```python
from build123d import *

# Parameters (mm, degrees)
F2_R     = 4.7625
F3_DEPTH = 9.525
F4_R     = 1.5875
F5_DEPTH = 22.225


with BuildPart() as f1:
    # F0 (on Front) → F1 (revolve)
    with BuildSketch(Plane.XZ):
        with BuildLine():
            Line((0, 60.744923), (0, 0))
            Line((0, 0), (13.365728, 15.209274))
            ThreePointArc((13.365728, 15.209274), (21.391858, 21.354408), (31.158879, 23.959541))
            ThreePointArc((31.158879, 23.959541), (20.775382, 29.638343), (8.941211, 29.773306))
            Line((8.941211, 29.773306), (7.487204, 29.773306))
            Line((7.487204, 29.773306), (7.837165, 60.744923))
            Line((7.837165, 60.744923), (0, 60.744923))
        make_face()
    revolve(axis=Axis((0, 0, 30.372461), (0, 0, -1)))

    # F2 (on face) → F3 (cut)
    with BuildSketch(Plane.XY.offset(60.744923)):
        Circle(F2_R)
    extrude(amount=-F3_DEPTH, mode=Mode.SUBTRACT)

    # F4 (on Top) → F5 (cut)
    with BuildSketch(Plane.XY):
        Circle(F4_R)
    extrude(amount=F5_DEPTH, mode=Mode.SUBTRACT)


solid = f1.part
```
Part model, mm, in its own coordinate system. A direction names the side the tool comes from. Give positions to 0.01 mm unless a question says otherwise; leave off trailing zeros. Order: outer loops, then holes, each group sorted by start corner. A loop starts at its lowest first (then second) coordinate and runs counter-clockwise, first axis right, second up. Notation, with made-up numbers: M 87,39 L 132,39 A28 ccw 132,61 Z; hole C 68,-34 d8. An arc over 180 degrees is marked long. Use a Markdown table: item, result. Add a question column.
(1) Drop flat-ended pins along their axis: P1, Ø5, axis at x = 8, z = 48.5, coming from the -Y side; P2, Ø1, axis at x = 0, y = 0, coming from the -Z side (3 decimals); P3, Ø3, axis at y = 17.5, z = 27, coming from the -X side. Give the stop position or say it passes through.
(2) Mould opens along Z. For faces 4 (the face through (3.54, 6.8, 45.48)), 5 (the face through (0, 5, 60.745)), 6 (the face through (-3.78, -2.9, 56.05)), 7 (the face through (0, 0, 22.225)) say: +Z half, -Z half, draft (parallel to the pull), parting line (faces both ways), or undercut.
(3) 3-axis set-ups, long thin cutter, end or side, ignore diameter. For faces 1 (the face through (0, 0, 51.22)), 2 (the face through (-0.34, -1.55, 11.87)), 3 (the face through (5, 6, 29.773)): which of +Z, -Z, +X, -X, +Y, -Y reach the whole face in a straight line?
(4) Saw through at A-A, the plane z = 20.5. Give the cut face in (x, y) (1 decimal), and give its area (3 significant figures).
(5) Saw through at C-C, the plane z = 12.5. Give the cut face in (x, y) (1 decimal).
(6) Saw through at B-B, the plane z = 36.5. Give the cut face in (x, y), and give its area (3 significant figures).
(7) Probe line 1 along X through (y, z) = (0, 11); line 2 along Y through (x, z) = (0, 57); line 3 along X through (y, z) = (0, 10.5). List the from-to ranges inside material, lowest first. Write a range as [from, to].
Answer key:
| question | item | result |
|---|---|---|
| 1 | P1 | y = -5.39 |
| 1 | P2 | z = 22.225 |
| 1 | P3 | x = -23.75 |
| 2 | face 4 | undercut |
| 2 | face 5 | +Z half |
| 2 | face 6 | draft |
| 2 | face 7 | -Z half |
| 3 | face 1 | +Z |
| 3 | face 2 | -Z |
| 3 | face 3 | none |
| 4 | outline | C 0,0 d39.6; hole C 0,0 d3.2 |
| 4 | area | 1,220 mm^2 |
| 5 | outline | C 0,0 d22; hole C 0,0 d3.2 |
| 6 | outline | C 0,0 d15.13 |
| 6 | area | 180 mm^2 |
| 7 | line 1 | [-9.67, -1.59], [1.59, 9.67] |
| 7 | line 2 | [-7.79, -4.76], [4.76, 7.79] |
| 7 | line 3 | [-9.23, -1.59], [1.59, 9.23] |
